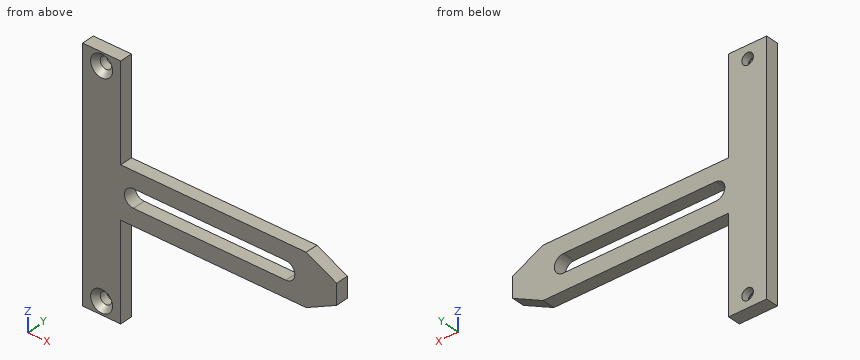
```python
from build123d import *

# Parameters (mm, degrees)
SKETCH2_W                                         = 63.5
SKETCH2_H                                         = 60.325
BOSS_EXTRUDE1_DEPTH                               = 1.5875
CUT_EXTRUDE1_REACH                                = 45.908
CUT_EXTRUDE2_REACH                                = 45.908
CSK_FOR_M2_5_FLAT_HEAD_MACHINE_SCREW1_D           = 2.9
CSK_FOR_M2_5_FLAT_HEAD_MACHINE_SCREW1_CSINK_D     = 5.5
CSK_FOR_M2_5_FLAT_HEAD_MACHINE_SCREW1_CSINK_ANGLE = 90


with BuildPart() as part:
    # Sketch2 → Boss-Extrude1 (new, symmetric)
    with BuildSketch(Plane(origin=(0, 0, 0), x_dir=(1, 0, 0), z_dir=(0, 1, 0))):
        Rectangle(SKETCH2_W, SKETCH2_H)
    extrude(amount=BOSS_EXTRUDE1_DEPTH, both=True)

    # Sketch4 → Cut-Extrude1 (cut, up to next)
    with BuildSketch(Plane(origin=(0, 1.5875, 0), x_dir=(1, 0, 0), z_dir=(0, 1, 0)), mode=Mode.PRIVATE) as cut_extrude1_sk1:
        Polygon((-22.225, -30.1625), (31.75, -30.1625), (31.75, -2.54), (24.13, -6.35), (-22.225, -6.35), align=None)
    cut_extrude1_tool1 = extrude(cut_extrude1_sk1.sketch, amount=-CUT_EXTRUDE1_REACH, mode=Mode.PRIVATE) & part.part
    # Sketch4 → Cut-Extrude1 (cut, up to next)
    with BuildSketch(Plane(origin=(0, 1.5875, 0), x_dir=(1, 0, 0), z_dir=(0, 1, 0)), mode=Mode.PRIVATE) as cut_extrude1_sk2:
        Polygon((31.75, 2.54), (24.13, 6.35), (-22.225, 6.35), (-22.225, 30.1625), (31.75, 30.1625), align=None)
    cut_extrude1_tool2 = extrude(cut_extrude1_sk2.sketch, amount=-CUT_EXTRUDE1_REACH, mode=Mode.PRIVATE) & part.part
    add(cut_extrude1_tool1.solids().sort_by_distance((5.035529, 1.5875, 18.109098))[0], mode=Mode.SUBTRACT)
    add(cut_extrude1_tool2.solids().sort_by_distance((5.035529, 1.5875, -18.109098))[0], mode=Mode.SUBTRACT)

    # Sketch5 → Cut-Extrude2 (cut, up to next)
    with BuildSketch(Plane(origin=(0, 1.5875, 0), x_dir=(1, 0, 0), z_dir=(0, 1, 0)), mode=Mode.PRIVATE) as cut_extrude2_sk1:
        with BuildLine():
            Line((-19.05, 2.2479), (19.05, 2.2479))
            ThreePointArc((19.05, 2.2479), (21.2979, 0), (19.05, -2.2479))
            Line((19.05, -2.2479), (-19.05, -2.2479))
            ThreePointArc((-19.05, -2.2479), (-21.2979, 0), (-19.05, 2.2479))
        make_face()
    cut_extrude2_tool1 = extrude(cut_extrude2_sk1.sketch, amount=-CUT_EXTRUDE2_REACH, mode=Mode.PRIVATE) & part.part
    add(cut_extrude2_tool1.solids().sort_by_distance((0, 1.5875, 0))[0], mode=Mode.SUBTRACT)

    # CSK for M2.5 Flat Head Machine Screw1 (through all)
    with Locations(Plane.XZ.offset(1.5875)):
        with Locations((-26.9875, 26.9875)):
            csk_for_m2_5_flat_head_machine_screw1 = CounterSinkHole(CSK_FOR_M2_5_FLAT_HEAD_MACHINE_SCREW1_D / 2, CSK_FOR_M2_5_FLAT_HEAD_MACHINE_SCREW1_CSINK_D / 2, counter_sink_angle=CSK_FOR_M2_5_FLAT_HEAD_MACHINE_SCREW1_CSINK_ANGLE)

    # Mirror1: CSK for M2.5 Flat Head Machine Screw1 across plane
    add(csk_for_m2_5_flat_head_machine_screw1.mirror(Plane.XY), mode=Mode.SUBTRACT)


solid = part.part
```
CAD build for the part. Positions are in the model's coordinates, mm. Round coordinates to 2 decimals unless told otherwise and drop trailing zeros. Loops run counter-clockwise (first coordinate to the right, second up) from the corner with the lowest first, then second, coordinate; pieces in that order, holes last. Notation, with made-up numbers: M -17,47 L -5,47 A10 ccw -5,59 Z; hole C 9,-1 d7. An arc over 180 degrees is marked long. Use a Markdown table: item, result. Add a question column.
(1) Cut at B-B (x = -18). Give the cut face in (y, z).
(2) Flat gauge pins, fed straight in: pin 1 (4 mm diameter, centred on x = -26.99, z = 26.99, fed in from +Y); pin 2 (1.6 mm diameter, centred on x = 11.5, y = 0.5, fed in from +Z); pin 3 (1 mm diameter, centred on x = -5.5, y = 1, fed in from -Z). Where does each tip first touch, or does it go through?
(3) Cut at C-C (y = -0.8). State how many separate pieces and enclosed holes the cut face has, and give its area (3 significant figures).
(4) Drill centre lines: line 1 (Z direction, x = -1, y = 0.3); line 2 (X direction, y = 0.75, z = -27) (3 decimals); line 3 (X direction, y = 0.55, z = 14.5) (3 decimals). Where is each one in solid material? Low to high.
(5) Cut at A-A (z = 0). Give the cut face in (x, y).
Geometry says:
| question | item | result |
|---|---|---|
| 1 | outline | M -1.59,-6.35 L 1.59,-6.35 L 1.59,-2.25 L -1.59,-2.25 Z; M -1.59,2.25 L 1.59,2.25 L 1.59,6.35 L -1.59,6.35 Z |
| 2 | pin 1 | stops at y = 1.59 |
| 2 | pin 2 | stops at z = 6.35 |
| 2 | pin 3 | stops at z = -6.35 |
| 3 | separate pieces | 1 |
| 3 | enclosed holes | 3 |
| 3 | area | 1,020 mm² |
| 4 | line 1 | z = -6.35 to -2.25, 2.25 to 6.35 |
| 4 | line 2 | x = -31.75 to -28.437, -25.538 to -22.225 |
| 4 | line 3 | x = -31.75 to -22.225 |
| 5 | outline | M -31.75,-1.59 L -21.3,-1.59 L -21.3,1.59 L -31.75,1.59 Z; M 21.3,-1.59 L 31.75,-1.59 L 31.75,1.59 L 21.3,1.59 Z |
